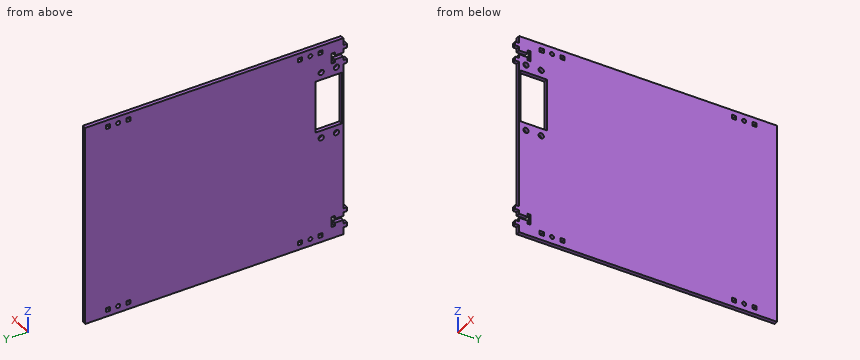
from build123d import *

# Parameters (mm, degrees)
BOSS_EXTRUDE2_DEPTH      = 1.5
BOSS_EXTRUDE2_DEPTH_BACK = 1.5
SKETCH1_R                = 1.575
SKETCH1_R_2              = 2.05
SKETCH1_W                = 40.5
SKETCH1_H                = 20.499999995
SKETCH1_W_2              = 3.15
SKETCH1_H_2              = 3.15


with BuildPart() as part:
    # Sketch1 → Boss-Extrude2 (new, two sides: drawn at the far end of the back side and taken through both)
    with BuildSketch(Plane(origin=(0, 0, 0), x_dir=(0, 0, -1), z_dir=(1, 0, 0)).offset(-BOSS_EXTRUDE2_DEPTH_BACK)):
        Polygon((11.425, 0), (8.5, 0), (8.5, -3), (5.5, -3), (5.5, 0), (0, 0), (0, 200), (156, 200), (156, 0), (150.5, 0), (150.5, -3), (147.5, -3), (147.5, 0), (144.575, 0), (144.575, 6.5), (147, 6.5), (147, 9), (139, 9), (139, 6.5), (141.425, 6.5), (141.425, 0), (138.5, 0), (138.5, -3), (135.5, -3), (135.5, 0), (20.5, 0), (20.5, -3), (17.5, -3), (17.5, 0), (14.575, 0), (14.575, 6.5), (17, 6.5), (17, 9), (9, 9), (9, 6.5), (11.425, 6.5), align=None)
        with Locations((5.25, 25.575)):
            Circle(SKETCH1_R, mode=Mode.SUBTRACT)
        with Locations(Location((5.25, 174.425, 0), (0, 0, 180))):
            Circle(SKETCH1_R, mode=Mode.SUBTRACT)
        with Locations((150.75, 174.425)):
            Circle(SKETCH1_R, mode=Mode.SUBTRACT)
        with Locations(Location((150.75, 25.575, 0), (0, 0, 180))):
            Circle(SKETCH1_R, mode=Mode.SUBTRACT)
        with Locations((73.2, 5.35)):
            Circle(SKETCH1_R_2, mode=Mode.SUBTRACT)
        with Locations((73.2, 17.149999995)):
            Circle(SKETCH1_R_2, mode=Mode.SUBTRACT)
        with Locations((21.2, 5.35)):
            Circle(SKETCH1_R_2, mode=Mode.SUBTRACT)
        with Locations((21.2, 17.149999995)):
            Circle(SKETCH1_R_2, mode=Mode.SUBTRACT)
        with Locations((47.2, 11.249999997)):
            Rectangle(SKETCH1_W, SKETCH1_H, mode=Mode.SUBTRACT)
        with Locations((5.25, 17.575)):
            Rectangle(SKETCH1_W_2, SKETCH1_H_2, mode=Mode.SUBTRACT)
        with Locations((5.25, 33.575)):
            Rectangle(SKETCH1_W_2, SKETCH1_H_2, mode=Mode.SUBTRACT)
        with Locations((5.25, 166.425)):
            Rectangle(SKETCH1_W_2, SKETCH1_H_2, mode=Mode.SUBTRACT)
        with Locations((5.25, 182.425)):
            Rectangle(SKETCH1_W_2, SKETCH1_H_2, mode=Mode.SUBTRACT)
        with Locations((150.75, 182.425)):
            Rectangle(SKETCH1_W_2, SKETCH1_H_2, mode=Mode.SUBTRACT)
        with Locations((150.75, 166.425)):
            Rectangle(SKETCH1_W_2, SKETCH1_H_2, mode=Mode.SUBTRACT)
        with Locations((150.75, 33.575)):
            Rectangle(SKETCH1_W_2, SKETCH1_H_2, mode=Mode.SUBTRACT)
        with Locations((150.75, 17.575)):
            Rectangle(SKETCH1_W_2, SKETCH1_H_2, mode=Mode.SUBTRACT)
    extrude(amount=BOSS_EXTRUDE2_DEPTH + BOSS_EXTRUDE2_DEPTH_BACK)


solid = part.part
Source: CAD feature listing. Evaluate the final solid. Frame: model axes, mm. Round coordinates to 2 decimals unless told otherwise and drop trailing zeros. Write each loop counter-clockwise with the first axis right and the second up, starting at its lowest first coordinate (ties: lowest second). Pieces come first, ordered by that corner, then holes. Notation, with made-up numbers: M 5,11 L 50,11 A31 ccw 50,50 Z; hole C 1,35.5 d5. An arc over 180 degrees is marked long. One line per item, written item: value. Start each with the question number.
Item 1: Section query A-A (z = -73.2). Return the cut outline in (x, y).
Item 2: Ray query, L1, parallel to Y at x = 0.8, z = -73; L2, parallel to Y at x = -0.6, z = -57.5; L3, parallel to Z at x = -1.05, y = 9.5. Return the intervals inside material, ascending. Write a range as from..to.
Item 3: Section query B-B (z = -46). Return the cut outline in (x, y).
Item 4: Section query C-C (x = 0.55). State how many separate pieces and enclosed holes the cut face has, plus the area to 3 significant figures.
Item 5: Pin query (flat end, axial travel): pin 1 (1.5 mm diameter, centred on x = 0.5, y = 34, fed in from +Z); pin 2 (1.5 mm diameter, centred on x = -0.5, y = -2, fed in from -Z). Return the tip coordinate at first contact, or that it passes through.
Result set:
1. outline: M -1.5,0 L 1.5,0 L 1.5,3.3 L -1.5,3.3 Z; M -1.5,7.4 L 1.5,7.4 L 1.5,15.1 L -1.5,15.1 Z; M -1.5,19.2 L 1.5,19.2 L 1.5,200 L -1.5,200 Z
2. L1: y = 0..3.31, 7.39..15.11, 19.19..200
2. L2: y = 0..1, 21.5..200
2. L3: z = -156..-67.45, -26.95..0
3. outline: M -1.5,0 L 1.5,0 L 1.5,1 L -1.5,1 Z; M -1.5,21.5 L 1.5,21.5 L 1.5,200 L -1.5,200 Z
4. separate pieces: 1
4. enclosed holes: 17
4. area: 30,200 mm²
5. pin 1: stops at z = 0
5. pin 2: stops at z = -150.5
